from build123d import *

# Parameters (mm, degrees)
SKETCH2_R          = 2.38125
CUT_EXTRUDE1_DEPTH = 10


with BuildPart() as part:
    # Sketch1 → Revolve1 (revolve)
    with BuildSketch(Plane.XY, mode=Mode.PRIVATE) as revolve1_sk:
        Polygon((-15.825, 13.7875), (-15.825, 11.6125), (-15.325, 11.1125), (2.675, 11.1125), (3.175, 11.6125), (3.175, 37.6), (2.675, 38.1), (0.5, 38.1), (0, 37.6), (0, 14.2875), (-15.325, 14.2875), align=None)
    revolve(revolve1_sk.sketch.rotate(Axis((0, 0, 0), (1, 0, 0)), 90), axis=Axis((0, 0, 0), (1, 0, 0)))

    # Sketch2 → Cut-Extrude1 (cut)
    with BuildSketch(Plane(origin=(3.175, 0, 0), x_dir=(0, 0, -1), z_dir=(1, 0, 0))):
        with Locations((-5.139303331, 31.331295238)):
            Circle(SKETCH2_R)
        with Locations((5.139303331, -31.331295238)):
            Circle(SKETCH2_R)
    extrude(amount=-CUT_EXTRUDE1_DEPTH, mode=Mode.SUBTRACT)


solid = part.part
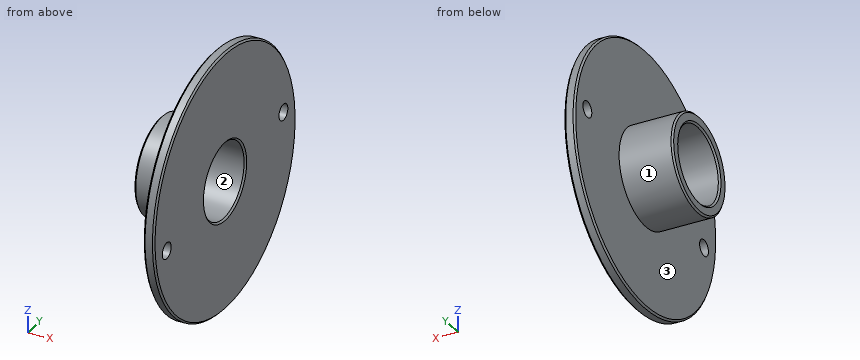
Source: CAD feature listing. Evaluate the final solid. Frame: model axes, mm. Face numbers are marked on the shaded views. Coordinates: 2 decimals unless noted, no trailing zeros. Order: outer loops, then holes, each group sorted by start corner. A loop starts at its lowest first (then second) coordinate and runs counter-clockwise, first axis right, second up. Notation, with made-up numbers: M -37,17.25 L 2,17.25 A16 cw 2,38.25 Z; hole C 77.25,88 d7. An arc over 180 degrees is marked long. Write each question's results on one line, items separated by ' | '. Start each with the question number.
1. Pin query (flat end, axial travel): pin 1 (3 mm diameter, centred on y = 31.33, z = 5.14, fed in from +X); pin 2 (5 mm diameter, centred on x = -1, z = 2, fed in from +Y); pin 3 (3 mm diameter, centred on x = -10.5, z = -2, fed in from +Y); pin 4 (1.5 mm diameter, centred on x = -6, y = -11.5, fed in from +Z). Return the tip coordinate at first contact, or that it passes through.
2. Section A-A, the plane y = 0. Return the cut outline in (x, z) (1 decimal), then the cut area to 3 significant figures.
3. Material intervals for L1, parallel to Y at x = -5, z = 0; L2, parallel to X at y = -21, z = 5 (3 decimals); L3, parallel to Z at x = -0.25, y = 9, sorted ascending.
4. Section C-C, the plane x = -7.25. Return the cut outline in (y, z) (1 decimal).
5. Draft query along Y for the marked faces 1, 2 and 3. Return one class per face: +Y half, -Y half, draft (parallel to the pull), parting line (faces both ways), or undercut.
Solution:
1) pin 1: through | pin 2: y = 38.1 | pin 3: y = 14.28 | pin 4: z = 9.41
2) outline: M -15.8,-13.8 L -15.3,-14.3 L 0,-14.3 L 0,-37.6 L 0.5,-38.1 L 2.7,-38.1 L 3.2,-37.6 L 3.2,-11.6 L 2.7,-11.1 L -15.3,-11.1 L -15.8,-11.6 Z; M -15.8,11.6 L -15.3,11.1 L 2.7,11.1 L 3.2,11.6 L 3.2,37.6 L 2.7,38.1 L 0.5,38.1 L 0,37.6 L 0,14.3 L -15.3,14.3 L -15.8,13.8 Z | area: 271 mm²
3) L1: -14.29 to -11.11, 11.11 to 14.29 | L2: 0 to 3.175 | L3: -11.1 to -6.52, 6.52 to 11.1
4) outline: C 0,0 d28.6; hole C 0,0 d22.2
5) face 1: parting line | face 2: undercut | face 3: draft
